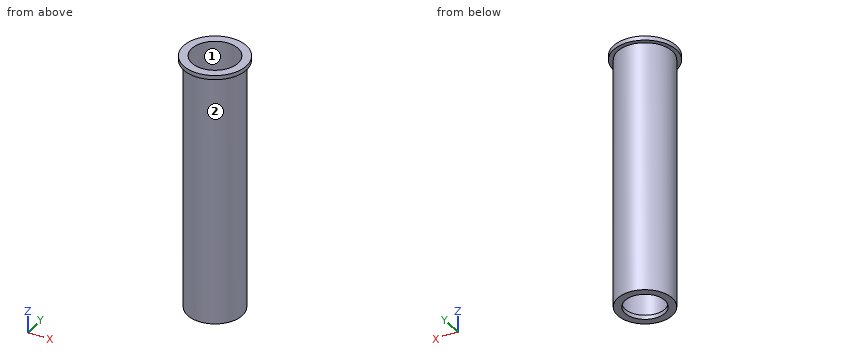
from build123d import *


with BuildPart() as part:
    # Croquis1 → Revolución1 (revolve)
    with BuildSketch(Plane.YZ, mode=Mode.PRIVATE) as revoluci_n1_sk:
        Polygon((11, -60), (11, 60), (15, 60), (15, 58), (13, 58), (13, -62), (9.5, -62), (9.5, -60), align=None)
    revolve(revoluci_n1_sk.sketch.rotate(Axis((0, 0, 0), (0, 0, 1)), 90), axis=Axis((0, 0, 0), (0, 0, 1)))


solid = part.part
Input: part model. Units: mm. Frame: model coordinates. Face numbers are marked on the shaded views. Round coordinates to 2 decimals unless told otherwise and drop trailing zeros. Order: outer loops, then holes, each group sorted by start corner. A loop starts at its lowest first (then second) coordinate and runs counter-clockwise, first axis right, second up. Notation, with made-up numbers: (-35, -1.5) - (6, -1.5) arc R23 cw to (6, 19.5) - close; hole circle Ø4 at (1, 20). An arc over 180 degrees is marked (long way). Answer as a JSON object with one key per item and string values. Group by question number.
(1) Cut plane A-A (y = 0). Return loops of the section in (x, z).
(2) Draft query along X for the marked faces 1 and 2. Return one class per face: released by +X, released by -X, zero draft, split by the parting line, or undercut.
(3) Material intervals for probe 1 along Y at (x, z) = (0, -60.6); probe 2 along Y at (x, z) = (0, -34); probe 3 along X at (y, z) = (-0.75, -48.5), sorted ascending. Write a range as from..to.
(4) Cut plane C-C (z = -33). Return loops of the section in (x, y), then the cut area to 3 significant figures.
(5) Pin query (flat end, axial travel): P1, Ø6.5, axis at x = 5, y = 0, coming from the +Z side; P2, Ø5, axis at y = 5, z = 31, coming from the -X side; P3, Ø1.5, axis at x = 3.5, z = -42, coming from the +Y side; P4, Ø1, axis at x = -9.5, z = -23, coming from the -Y side. Return the tip coordinate at first contact, or that it passes through.
Here are the results:
{
 "1": {"outline": "(-15, 58) - (-13, 58) - (-13, -62) - (-9.5, -62) - (-9.5, -60) - (-11, -60) - (-11, 60) - (-15, 60) - close; (9.5, -62) - (13, -62) - (13, 58) - (15, 58) - (15, 60) - (11, 60) - (11, -60) - (9.5, -60) - close"},
 "2": {"face 1": "undercut", "face 2": "split by the parting line"},
 "3": {"probe 1": "y = -13..-9.5, 9.5..13", "probe 2": "y = -13..-11, 11..13", "probe 3": "x = -12.98..-10.97, 10.97..12.98"},
 "4": {"outline": "circle Ø26 at (0, 0); hole circle Ø22 at (0, 0)", "area": "151 mm^2"},
 "5": {"P1": "passes through", "P2": "stops at x = -12.76", "P3": "stops at y = 12.71", "P4": "stops at y = -9.38"}
}
